Part model, mm, in its own coordinate system. Face numbers are marked on the shaded views. Coordinates: 2 decimals unless noted, no trailing zeros. Loops run counter-clockwise (first coordinate to the right, second up) from the corner with the lowest first, then second, coordinate; pieces in that order, holes last. Notation, with made-up numbers: (-1.5, 6) - (42.5, 6) arc R28 cw to (42.5, 26) - close; hole circle Ø11 at (45, 4.25). An arc over 180 degrees is marked (long way). Use a Markdown table: item, result. Add a question column.
1. Band-saw the part on A-A, the plane y = -9. Give the cut face in (x, z) (3 decimals), plus the area to 3 significant figures.
2. Pull direction X, two halves, no side cores. Call the marked faces 1 and 2: pulls with the +X half, pulls with the -X half, needs draft (parallel to the pull), parting line crosses it, or undercut.
3. Wall check: probe 1 along X at (y, z) = (0, 41) (3 decimals); probe 2 along Y at (x, z) = (15.5, 20) (3 decimals). Give the ranges that are in metal, low to high. Write a range as [from, to].
4. Band-saw the part on C-C, the plane x = -5. Give the cut face in (y, z) (3 decimals).
5. Band-saw the part on B-B, the plane z = 440.5. Give the cut face in (x, y) (3 decimals), plus the area to 3 significant figures.
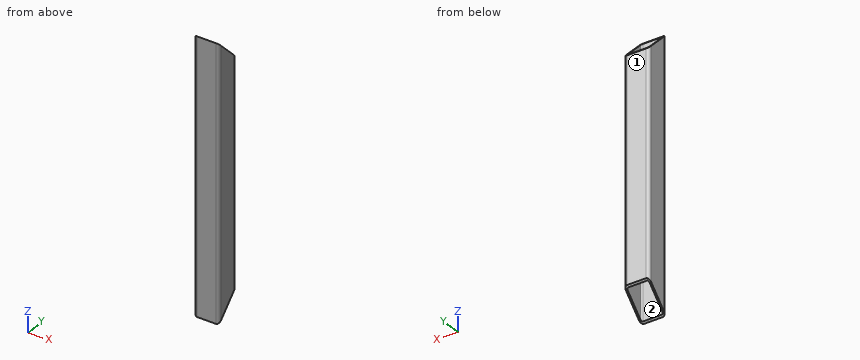
Autodesk Inventor part; units mm, degrees
ref_plane "Start Plane" through (0, 0, -25.4) normal (0, 0, 1) x (1, 0, 0)
ref_plane "End Plane" through (0, 0, 533.4) normal (0, 0, 1) x (1, 0, 0)
ref_plane "Work Plane4" through (0, -25.4, -25.4) normal (0, 0.7071, -0.7071) x (1, 0, 0)
ref_plane "Start Plane" through (0, 0, -25.4) normal (0, 0, 1) x (1, 0, 0)
ref_plane "End Plane" through (0, 0, 533.4) normal (0, 0, 1) x (1, 0, 0)
sketch "Sketch" plane through (0, 0, 0) normal (0, 0, 1) x (1, 0, 0)
  line L0 (-25.4, -19.05) -> (-25.4, 19.05)
  line L1 (-19.05, 25.4) -> (19.05, 25.4)
  line L2 (25.4, 19.05) -> (25.4, -19.05)
  line L3 (19.05, -25.4) -> (-19.05, -25.4)
  arc A0 (-25.4, -19.05) -> (-19.05, -25.4) centre (-19.05, -19.05) ccw
  arc A1 (-19.05, 25.4) -> (-25.4, 19.05) centre (-19.05, 19.05) ccw
  arc A2 (25.4, 19.05) -> (19.05, 25.4) centre (19.05, 19.05) ccw
  arc A3 (19.05, -25.4) -> (25.4, -19.05) centre (19.05, -19.05) ccw
  arc A4 (-19.05, 22.225) -> (-22.225, 19.05) centre (-19.05, 19.05) ccw
  line L4 (-19.05, 22.225) -> (19.05, 22.225)
  arc A5 (22.225, 19.05) -> (19.05, 22.225) centre (19.05, 19.05) ccw
  line L5 (22.225, 19.05) -> (22.225, -19.05)
  arc A6 (19.05, -22.225) -> (22.225, -19.05) centre (19.05, -19.05) ccw
  line L6 (19.05, -22.225) -> (-19.05, -22.225)
  arc A7 (-22.225, -19.05) -> (-19.05, -22.225) centre (-19.05, -19.05) ccw
  line L7 (-22.225, -19.05) -> (-22.225, 19.05)
  line L8 (0, 37.4012) -> (0, -37.4012) construction
  line L9 (-37.4012, 0) -> (37.4012, 0) construction
  dimension "d10" = 50.8
  dimension "d11" = 50.8
  dimension "d12" = 3.175
  dimension "d15" = 25.4
  dimension "d16" = 25.4
  dimension "d17" = 6.35
extrude "Body" add sketch "Sketch" along normal up to surface (558.8 mm away) from surface at -25.4
sketch "Sketch3" plane through (0, 0, 0) normal (0, 0, 1) x (1, 0, 0)
  line L0 (0, 0) -> (10, 0)
ref_plane "Work Plane3" through (0, 0, 0) normal (0, -1, 0) x (1, 0, 0)
sketch "Sketch4" plane through (0, 0, 0) normal (0, -1, 0) x (1, 0, 0)
  line L0 (-2, -25.4) -> (12, -25.4)
  line L1 (-2, 533.4) -> (12, 533.4)
  dimension "d19" = 558.8
ref_plane "Work Plane4" through (0, -25.4, -25.4) normal (0, 0.7071, -0.7071) x (1, 0, 0)
split "Split1" plane through (0, -25.4, -25.4) removes the side toward (0, 0.7071, -0.7071)
ref_plane "Work Plane5" through (0, -25.4, 533.4) normal (0, 0.7071, 0.7071) x (1, 0, 0)
split "Split2" plane through (0, -25.4, 533.4) removes the side toward (0, 0.7071, 0.7071)
equation "\"d10\" = G_H"
equation "\"d11\" = G_W"
equation "\"d12\" = G_T"
equation "\"d15\" = 0.5 * d10"
equation "\"d16\" = 0.5 * d11"
equation "\"d17\" = G_IR"
equation "\"d3\" = G_L"
equation "\"G_W\" = 50.8"
equation "\"G_H\" = 50.8"
equation "\"G_T\" = 3.175"
equation "\"G_IR\" = 6.35"
equation "\"G_L\" = d19"
equation "\"G_OFFSET_START\" = 25.4"
equation "\"G_OFFSET_END\" = 25.4"
equation "\"d13\" = -G_OFFSET_START"
equation "\"d14\" = G_OFFSET_END + B_L"
equation "\"B_L\" = 508"
properties part number "AISC - 2 x 2 x 1/8 - 22" material "Steel, Mild"
Geometry check:
| question | item | result |
|---|---|---|
| 1 | outline | (-25.4, -9) - (-22.225, -9) - (-22.225, 517) - (-25.4, 517) - close; (22.225, -9) - (25.4, -9) - (25.4, 517) - (22.225, 517) - close |
| 1 | area | 3,340 mm^2 |
| 2 | face 1 | needs draft |
| 2 | face 2 | undercut |
| 3 | probe 1 | x = [-25.4, -22.225], [22.225, 25.4] |
| 3 | probe 2 | y = [-25.4, -22.225] |
| 4 | outline | (-25.4, -25.4) - (-22.225, -22.225) - (-22.225, 530.225) - (-25.4, 533.4) - close; (22.225, 22.225) - (25.4, 25.4) - (25.4, 482.6) - (22.225, 485.775) - close |
| 5 | outline | (-25.4, -19.05) arc R6.35 ccw to (-19.05, -25.4) - (19.05, -25.4) arc R6.35 ccw to (25.4, -19.05) - (25.4, 19.05) arc R6.35 ccw to (19.05, 25.4) - (-19.05, 25.4) arc R6.35 ccw to (-25.4, 19.05) - close; hole (-22.225, -19.05) arc R3.175 ccw to (-19.05, -22.225) - (19.05, -22.225) arc R3.175 ccw to (22.225, -19.05) - (22.225, 19.05) arc R3.175 ccw to (19.05, 22.225) - (-19.05, 22.225) arc R3.175 ccw to (-22.225, 19.05) - close |
| 5 | area | 579 mm^2 |
